Build history of the part. All positions in model axes, mm. Face numbers are marked on the shaded views. A direction names the side the tool comes from. Coordinates: 2 decimals unless noted, no trailing zeros. Write each loop counter-clockwise with the first axis right and the second up, starting at its lowest first coordinate (ties: lowest second). Pieces come first, ordered by that corner, then holes. Notation, with made-up numbers: (27, -18) -> (34, -18) arc R13 cw to (34, -3) -> close; hole circle Ø2 at (1.25, 8). An arc over 180 degrees is marked (long way). Write each question's results on one line, items separated by ' | '. Start each with the question number.
Q1. Saw through at C-C on x = 78. Give the cut face in (y, z) (3 decimals).
Q2. Saw through at A-A on z = 1.75. Give the cut face in (x, y) (1 decimal).
Q3. Saw through at D-D on z = -9. Give the cut face in (x, y) (1 decimal), and give its area (3 significant figures).
Q4. Drill centre lines: line 1 (X direction, y = 4, z = 2.5); line 2 (X direction, y = -1.5, z = -9.25); line 3 (X direction, y = 2.75, z = -5.5). Where is each one in solid material? Low to high.
Q5. Drop flat-ended pins along their axis: pin 1 Ø1.6 at (x, z) = (8, -1.5) entering from -Y; pin 2 Ø1 at (x, z) = (8, 0) entering from +Y (3 decimals); pin 3 Ø3 at (y, z) = (-8, 1) entering from -X; pin 4 Ø2 at (x, y) = (8, -0.5) entering from +Z. Give the stop position or say it passes through.
Q6. Saw through at B-B on y = 4.5. Give the cut face in (x, z) (3 decimals), and give its area (3 significant figures).
Q7. Tool access for the marked faces 1 and 2: list every direction of +Z, -Z, +X, -X, +Y, -Y with a clear straight run to the whole face (end or side of a thin tool).
from build123d import *

# Parameters (mm, degrees)
SKETCH1_R               = 7.1501
BOSS_EXTRUDE1_DEPTH     = 4.7498
SKETCH1_R_2             = 11.1125
SKETCH1_R_3             = 5.5626
BOSS_EXTRUDE1_2_DEPTH   = 4.7498
BOSS_EXTRUDE2_DEPTH     = 11.1252
BOSS_EXTRUDE3_START     = -15.875
SKETCH1_4_R             = 11.1125
SKETCH1_4_R_2           = 5.5626
SKETCH1_4_R_3           = 7.1501
BOSS_EXTRUDE3_DEPTH     = 15.875
CUT_EXTRUDE2_DEPTH      = 4.826
CUT_EXTRUDE2_DEPTH_BACK = 4.6736


with BuildPart() as part:
    # Sketch1 → Boss-Extrude1 (new body)
    with BuildSketch(Plane.XY):
        with BuildLine():
            Line((1.188561525, 14.237976603), (0, 14.2875))
            ThreePointArc((0, 14.2875), (-14.2875, 0), (0, -14.2875))
            Line((0, -14.2875), (1.188561525, -14.237976603))
            ThreePointArc((1.188561525, -14.237976603), (10.514614331, -9.673445184), (14.2875, 0))
            ThreePointArc((14.2875, 0), (10.514614331, 9.673445184), (1.188561525, 14.237976603))
        make_face()
        Circle(SKETCH1_R, mode=Mode.SUBTRACT)
    extrude(amount=BOSS_EXTRUDE1_DEPTH)



with BuildPart() as body_2:
    # Sketch1 → Boss-Extrude1 2 (new body)
    with BuildSketch(Plane.XY):
        with Locations((76.2, 0)):
            Circle(SKETCH1_R_2)
        with Locations((76.2, 0)):
            Circle(SKETCH1_R_3, mode=Mode.SUBTRACT)
    extrude(amount=BOSS_EXTRUDE1_2_DEPTH)


with BuildPart() as body_3:
    # Sketch1_3 → Boss-Extrude2 (new body)
    with BuildSketch(Plane.XY):
        with BuildLine():
            Line((76.2, 11.1125), (1.188561525, 14.237976603))
            ThreePointArc((1.188561525, 14.237976603), (10.514614331, 9.673445184), (14.2875, 0))
            ThreePointArc((14.2875, 0), (10.514614331, -9.673445184), (1.188561525, -14.237976603))
            Line((1.188561525, -14.237976603), (76.2, -11.1125))
            ThreePointArc((76.2, -11.1125), (65.0875, 0), (76.2, 11.1125))
        make_face()
    extrude(amount=-BOSS_EXTRUDE2_DEPTH)


with BuildPart() as part_1:
    add(part.part)

    add(body_2.part)  # Boss-Extrude3 merges body 2

    add(body_3.part)  # Boss-Extrude3 merges body 3
    # Sketch1_4 → Boss-Extrude3 (add)
    # profile 1 of 2: a face of its own
    with BuildSketch(Plane.XY.offset(BOSS_EXTRUDE3_START)):
        with Locations((76.2, 0)):
            Circle(SKETCH1_4_R)
        with Locations((76.2, 0)):
            Circle(SKETCH1_4_R_2, mode=Mode.SUBTRACT)
    # profile 2 of 2: a face of its own
    with BuildSketch(Plane.XY.offset(BOSS_EXTRUDE3_START)):
        with BuildLine():
            Line((1.188561525, 14.237976603), (0, 14.2875))
            ThreePointArc((0, 14.2875), (-14.2875, 0), (0, -14.2875))
            Line((0, -14.2875), (1.188561525, -14.237976603))
            ThreePointArc((1.188561525, -14.237976603), (10.514614331, -9.673445184), (14.2875, 0))
            ThreePointArc((14.2875, 0), (10.514614331, 9.673445184), (1.188561525, 14.237976603))
        make_face()
        Circle(SKETCH1_4_R_3, mode=Mode.SUBTRACT)
    extrude(amount=BOSS_EXTRUDE3_DEPTH)

    # Sketch2 → Cut-Extrude2 (cut, two sides: drawn at the far end of the back side and taken through both)
    with BuildSketch(Plane.XY.offset(-CUT_EXTRUDE2_DEPTH_BACK)):
        Polygon((6.971640679, 0), (6.971640679, 1.5875), (8.927440679, 1.5875), (8.927440679, -1.5875), (6.971640679, -1.5875), align=None)
    extrude(amount=CUT_EXTRUDE2_DEPTH + CUT_EXTRUDE2_DEPTH_BACK, mode=Mode.SUBTRACT)


solid = part_1.part
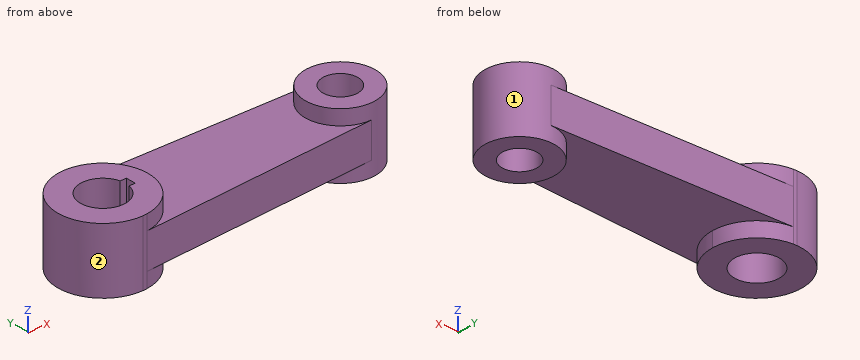
Returned:
1) outline: (-10.966, -15.875) -> (-5.263, -15.875) -> (-5.263, 4.75) -> (-10.966, 4.75) -> close; (5.263, -15.875) -> (10.966, -15.875) -> (10.966, 4.75) -> (5.263, 4.75) -> close
2) outline: (0, -14.3) -> (1.2, -14.2) arc R14.3 ccw to (1.2, 14.2) -> (0, 14.3) arc R14.3 ccw to start; circle Ø22.2 at (76.2, 0); hole (7, -1.6) -> (8.9, -1.6) -> (8.9, 1.6) -> (7, 1.6) arc R7.2 ccw (long way) to start; hole circle Ø11.1 at (76.2, 0)
3) outline: (0, -14.3) -> (76.2, -11.1) arc R11.1 ccw to (76.2, 11.1) -> (0, 14.3) arc R14.3 ccw to start; hole circle Ø14.3 at (0, 0); hole circle Ø11.1 at (76.2, 0) | area: 2,190 mm2
4) line 1: x = -13.72 to -5.93, 5.93 to 13.72, 65.83 to 72.33, 80.07 to 86.57 | line 2: x = -14.21 to -6.99, 6.99 to 70.84, 81.56 to 87.21 | line 3: x = -14.02 to -6.6, 6.6 to 71.36, 81.04 to 86.97
5) pin 1: stops at y = -13.99 | pin 2: stops at y = 13.975 | pin 3: stops at x = -12.72 | pin 4: stops at z = 4.75
6) outline: (-13.56, -15.875) -> (-5.556, -15.875) -> (-5.556, 4.75) -> (-13.56, 4.75) -> close; (5.556, -15.875) -> (13.56, -15.875) -> (13.56, -11.125) -> (66.039, -11.125) -> (66.039, -15.875) -> (72.93, -15.875) -> (72.93, 4.75) -> (66.039, 4.75) -> (66.039, 0) -> (13.56, 0) -> (13.56, 4.75) -> (5.556, 4.75) -> close; (79.47, -15.875) -> (86.361, -15.875) -> (86.361, 4.75) -> (79.47, 4.75) -> close | area: 1,200 mm2
7) face 1: none | face 2: +Z, -Z, -X
